CAD build for the part. Positions are in the model's coordinates, mm. Face numbers are marked on the shaded views. A direction names the side the tool comes from. Coordinates: 2 decimals unless noted, no trailing zeros. Order: outer loops, then holes, each group sorted by start corner. A loop starts at its lowest first (then second) coordinate and runs counter-clockwise, first axis right, second up. Notation, with made-up numbers: M -10.75,80.5 L -0.75,80.5 A28 cw -0.75,116.5 Z; hole C 32.5,37.25 d11. An arc over 180 degrees is marked long. Write item = value, one per line.
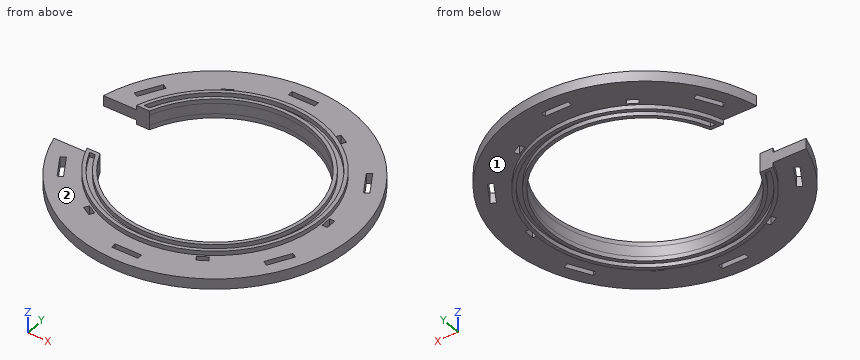
Autodesk Inventor part; units mm, degrees
ref_plane "YZ Plane" through (0, 0, 0) normal (1, 0, 0) x (0, 1, 0)
ref_plane "XZ Plane" through (0, 0, 0) normal (0, 1, 0) x (-1, 0, 0)
ref_plane "XY Plane" through (0, 0, 0) normal (0, 0, 1) x (1, 0, 0)
sketch "Sketch1" plane through (0, 0, 0) normal (0, 0, 1) x (1, 0, 0)
  circle A0 centre (0, 0) radius 80
  circle A1 centre (0, 0) radius 55
  line L0 (-7.5, 73) -> (7.5, 73)
  line L1 (7.5, 73) -> (7.5, 70)
  line L2 (7.5, 70) -> (-7.5, 70)
  line L3 (-7.5, 70) -> (-7.5, 73)
  line L4 (-66.9699, 30.0048) -> (-59.4699, 42.9952)
  line L5 (-59.4699, 42.9952) -> (-56.8718, 41.4952)
  line L6 (-56.8718, 41.4952) -> (-64.3718, 28.5048)
  line L7 (-64.3718, 28.5048) -> (-66.9699, 30.0048)
  line L8 (-59.4699, -42.9952) -> (-66.9699, -30.0048)
  line L9 (-66.9699, -30.0048) -> (-64.3718, -28.5048)
  line L10 (-64.3718, -28.5048) -> (-56.8718, -41.4952)
  line L11 (-56.8718, -41.4952) -> (-59.4699, -42.9952)
  line L12 (7.5, -73) -> (-7.5, -73)
  line L13 (-7.5, -73) -> (-7.5, -70)
  line L14 (-7.5, -70) -> (7.5, -70)
  line L15 (7.5, -70) -> (7.5, -73)
  line L16 (66.9699, -30.0048) -> (59.4699, -42.9952)
  line L17 (59.4699, -42.9952) -> (56.8718, -41.4952)
  line L18 (56.8718, -41.4952) -> (64.3718, -28.5048)
  line L19 (64.3718, -28.5048) -> (66.9699, -30.0048)
  line L20 (59.4699, 42.9952) -> (66.9699, 30.0048)
  line L21 (66.9699, 30.0048) -> (64.3718, 28.5048)
  line L22 (64.3718, 28.5048) -> (56.8718, 41.4952)
  line L23 (56.8718, 41.4952) -> (59.4699, 42.9952)
  line L24 (-58.1708, 43.7452) -> (-43.1708, 43.7452)
  line L25 (-43.1708, 43.7452) -> (-43.1708, 40.7452)
  line L26 (-43.1708, 40.7452) -> (-58.1708, 40.7452)
  line L27 (-58.1708, 40.7452) -> (-58.1708, 43.7452)
  line L28 (-58.1708, -40.7452) -> (-43.1708, -40.7452)
  line L29 (-43.1708, -40.7452) -> (-43.1708, -43.7452)
  line L30 (-43.1708, -43.7452) -> (-58.1708, -43.7452)
  line L31 (-58.1708, -43.7452) -> (-58.1708, -40.7452)
  line L32 (0, 20) -> (-100, 20)
  line L33 (-100, 20) -> (-100, -20)
  line L34 (-100, -20) -> (0, -20)
  line L35 (0, -20) -> (0, 20)
  point P0 (0, 73)
  point P1 (7.5, 71.5)
  point P2 (0, 70)
  point P3 (-63.2199, 36.5)
  point P4 (-58.1708, 42.2452)
  point P5 (-60.6218, 35)
  point P6 (-63.2199, -36.5)
  point P7 (-65.6708, -29.2548)
  point P8 (-60.6218, -35)
  point P9 (0, -73)
  point P10 (-7.5, -71.5)
  point P11 (0, -70)
  point P12 (63.2199, -36.5)
  point P13 (58.1708, -42.2452)
  point P14 (60.6218, -35)
  point P15 (63.2199, 36.5)
  point P16 (65.6708, 29.2548)
  point P17 (60.6218, 35)
  point P18 (-58.1708, 42.2452)
  point P19 (-58.1708, -42.2452)
  point P20 (-51.2348, -20)
  point P21 (-77.4597, -20)
  point P22 (-77.4597, 20)
  point P23 (-51.2348, 20)
  dimension "d0" = 160
  dimension "d1" = 110
  dimension "d2" = 15
  dimension "d3" = 3
  dimension "d11" = 70
  dimension "d14" = 360
  dimension "d18" = 15
  dimension "d19" = 3
  dimension "d20" = 15
  dimension "d21" = 3
  dimension "d22" = 40
  dimension "d23" = 100
extrude "Extrusion2" add sketch "Sketch1" along normal blind 6 contours A0 L34 A1 L32 | L27 L24 L25 L26 L6 L5 | L11 L10 L28 L29 L30 L31 picked at (16.7927, -65.9701)
sketch "草圖2" plane through (0, 0, 6) normal (0, 0, 1) x (1, 0, 0)
  arc A0 (-51.2348, -20) -> (-51.2348, 20) centre (0, 0) ccw
  circle A1 centre (0, 0) radius 55
  circle A2 centre (0, 0) radius 57
  circle A3 centre (0, 0) radius 60
  circle A4 centre (0, 0) radius 62
  arc A5 (-77.4597, -20) -> (-77.4597, 20) centre (0, 0) ccw
  line L0 (-51.2348, 20) -> (-77.4597, 20)
  line L1 (-51.2348, -20) -> (-77.4597, -20)
  line L2 (-51.2348, -20) -> (-77.4597, -20)
  line L3 (-51.2348, 20) -> (-77.4597, 20)
  line L4 (-77.4597, 20) -> (-77.4597, 22)
  line L5 (-77.4597, 22) -> (-51.2348, 22)
  line L6 (-51.2348, 22) -> (-51.2348, 20)
  line L7 (-77.4597, -20) -> (-51.2348, -20)
  line L8 (-51.2348, -20) -> (-51.2348, -22)
  line L9 (-51.2348, -22) -> (-77.4597, -22)
  line L10 (-77.4597, -22) -> (-77.4597, -20)
  point P0 (-58.6856, 20)
  point P1 (-58.6856, -20)
  point P2 (-55.8211, 22)
  point P3 (-55.8211, -22)
  point P4 (-52.5833, -22)
  point P5 (-52.5833, 22)
  dimension "d24" = 114
  dimension "d25" = 120
  dimension "d26" = 124
  dimension "d27" = 2
  dimension "d28" = 26.2249
  dimension "d29" = 2
  dimension "d30" = 26.2249
extrude "擠出3" add sketch "草圖2" against normal blind 8.5 contours L8 L9 A2 L1 | A0 L6 L5 A2 L9 L8 | L0 A2 L5 L6 | A2 L9 A3 L1 | L0 A3 L5 A2 | A3 L9 A4 L1 | L0 A4 L5 A3 | A3 L5 A4 L9
extrude "擠出4" add sketch "草圖2" along normal blind 2.5 contours L8 L9 A2 L1 | A0 L6 L5 A2 L9 L8 | L0 A2 L5 L6 | A2 L9 A3 L1 | L0 A3 L5 A2 | A3 L9 A4 L1 | L0 A4 L5 A3 | A3 L5 A4 L9
sketch "草圖3" plane through (0, 0, 6) normal (0, 0, 1) x (1, 0, 0)
  line L0 (63, 3) -> (66, 3)
  line L1 (66, 3) -> (66, -3)
  line L2 (66, -3) -> (63, -3)
  line L3 (63, -3) -> (63, 3)
  line L4 (28.9019, 56.0596) -> (30.4019, 58.6577)
  line L5 (30.4019, 58.6577) -> (35.5981, 55.6577)
  line L6 (35.5981, 55.6577) -> (34.0981, 53.0596)
  line L7 (34.0981, 53.0596) -> (28.9019, 56.0596)
  line L8 (-34.0981, 53.0596) -> (-35.5981, 55.6577)
  line L9 (-35.5981, 55.6577) -> (-30.4019, 58.6577)
  line L10 (-30.4019, 58.6577) -> (-28.9019, 56.0596)
  line L11 (-28.9019, 56.0596) -> (-34.0981, 53.0596)
  line L12 (-63, -3) -> (-66, -3)
  line L13 (-66, -3) -> (-66, 3)
  line L14 (-66, 3) -> (-63, 3)
  line L15 (-63, 3) -> (-63, -3)
  line L16 (-28.9019, -56.0596) -> (-30.4019, -58.6577)
  line L17 (-30.4019, -58.6577) -> (-35.5981, -55.6577)
  line L18 (-35.5981, -55.6577) -> (-34.0981, -53.0596)
  line L19 (-34.0981, -53.0596) -> (-28.9019, -56.0596)
  line L20 (34.0981, -53.0596) -> (35.5981, -55.6577)
  line L21 (35.5981, -55.6577) -> (30.4019, -58.6577)
  line L22 (30.4019, -58.6577) -> (28.9019, -56.0596)
  line L23 (28.9019, -56.0596) -> (34.0981, -53.0596)
  point P0 (0, 0)
  point P1 (63, 0)
  point P2 (31.5, 54.5596)
  point P3 (-31.5, 54.5596)
  point P4 (-63, 0)
  point P5 (-31.5, -54.5596)
  point P6 (31.5, -54.5596)
  dimension "d42" = 3
  dimension "d43" = 6
  dimension "d44" = 63
  dimension "d47" = 360
extrude "擠出5" cut sketch "草圖3" against normal through all contours L0 L1 L2 L3 | L4 L5 L6 L7 | L8 L9 L10 L11 | L16 L17 L18 L19 | L20 L21 L22 L23
properties part number "[3DP]back_cir_hold_final" material "MDF Medium Density Fiberboard"
(1) Pin check, flat tips, straight feed: pin 1 Ø3 at (y, z) = (-0.5, 4.5) entering from +X; pin 2 Ø6 at (y, z) = (33.5, 1) entering from -X; pin 3 Ø6 at (x, y) = (41, 53) entering from -Z. Stop position of each tip, or through.
Evaluation:
pin_1 = 80
pin_2 = -73.96
pin_3 = 0
(2) Wall check: line 1 (Y direction, x = 0, z = -1); line 2 (X direction, y = 32, z = 5); line 3 (X direction, y = 57.5, z = 5.25). Give the ranges that are in metal, low to high. Write a range as from..to.
Evaluation:
line_1 = -62..-60, -57..-55, 55..57, 60..62
line_2 = -73.32..-65.82, -62.35..-44.73, 44.73..62.35, 65.82..73.32
line_3 = -55.62..-32.41, -29.73..29.73, 32.41..55.62
(3) Slice it at A-A, the plane y = 0. Write the cut outline in (x, z).
Evaluation:
outline = M 55,-2.5 L 57,-2.5 L 57,0 L 60,0 L 60,-2.5 L 62,-2.5 L 62,0 L 63,0 L 63,6 L 62,6 L 62,8.5 L 60,8.5 L 60,6 L 57,6 L 57,8.5 L 55,8.5 L 55,6 Z; M 66,0 L 80,0 L 80,6 L 66,6 Z
(4) Tool access for the marked faces 1 and 2: list every direction of +Z, -Z, +X, -X, +Y, -Y with a clear straight run to the whole face (end or side of a thin tool).
Evaluation:
face_1 = -Z
face_2 = +Z
(5) Slice it at B-B, the plane x = 0. State how many separate pieces and enclosed holes the cut face has, then the cut area to 3 significant figures.
Evaluation:
separate_pieces = 4
enclosed_holes = 0
area = 304 mm²
